from build123d import *

# Parameters (mm, degrees)
SKETCH_1_R      = 1.75
EXTRUDE_1_DEPTH = 1.6
SKETCH_2_W      = 61.5
SKETCH_2_H      = 44.5
EXTRUDE_2_DEPTH = 5.2


with BuildPart() as part:
    # 草图1 → 凸台-拉伸1 (new body)
    with BuildSketch(Plane(origin=(0, 0, 0), x_dir=(1, 0, 0), z_dir=(0, 1, 0))):
        with BuildLine():
            Line((1.5, 0), (73, 0))
            ThreePointArc((73, 0), (74.060660172, 0.439339828), (74.5, 1.5))
            Line((74.5, 1.5), (74.5, 41.5))
            ThreePointArc((74.5, 41.5), (74.060660172, 42.560660172), (73, 43))
            Line((73, 43), (1.5, 43))
            ThreePointArc((1.5, 43), (0.439339828, 42.560660172), (0, 41.5))
            Line((0, 41.5), (0, 1.5))
            ThreePointArc((0, 1.5), (0.439339828, 0.439339828), (1.5, 0))
        make_face()
        with Locations(Location((3.05, 39.85, 0), (0, 0, 270))):
            Circle(SKETCH_1_R, mode=Mode.SUBTRACT)
        with Locations(Location((3.05, 3.15, 0), (0, 0, 270))):
            Circle(SKETCH_1_R, mode=Mode.SUBTRACT)
        with Locations(Location((71.45, 39.85, 0), (0, 0, 270))):
            Circle(SKETCH_1_R, mode=Mode.SUBTRACT)
        with Locations(Location((71.45, 3.15, 0), (0, 0, 270))):
            Circle(SKETCH_1_R, mode=Mode.SUBTRACT)
    extrude(amount=EXTRUDE_1_DEPTH)

    # 草图2 → 凸台-拉伸2 (add)
    with BuildSketch(Plane(origin=(0, 1.6, 0), x_dir=(1, 0, 0), z_dir=(0, 1, 0))):
        with Locations((37.25, 21.5)):
            Rectangle(SKETCH_2_W, SKETCH_2_H)
    extrude(amount=EXTRUDE_2_DEPTH)


solid = part.part
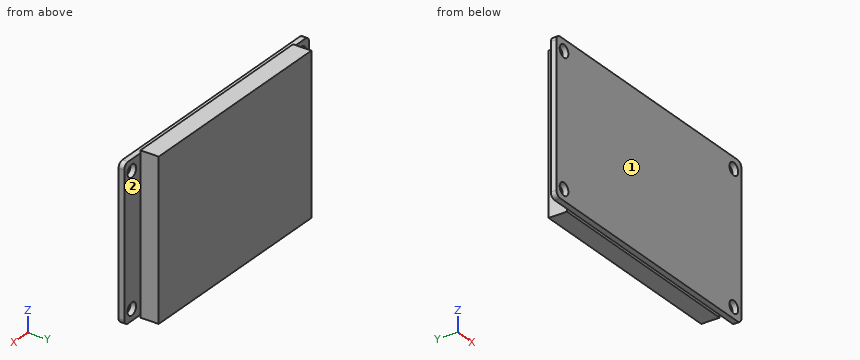
The listing builds one solid part. Answer for the finished solid, in the listing's coordinates (mm). Face numbers are marked on the shaded views. A direction names the side the tool comes from. Give positions to 0.01 mm unless a question says otherwise; leave off trailing zeros. Loops run counter-clockwise (first coordinate to the right, second up) from the corner with the lowest first, then second, coordinate; pieces in that order, holes last. Notation, with made-up numbers: M -9,-18 L 7,-18 A23 ccw 7,21 Z; hole C -23,31.5 d11. An arc over 180 degrees is marked long. Answer as CSV lines item,"result".
Item 1: The part is cut by section D-D (y = 3.5). Give the vertices of the cut face in (x, z).
Values follow:
outline,"M 6.5,-43.75 L 68,-43.75 L 68,0.75 L 6.5,0.75 Z"
Item 2: The part is cut by section C-C (z = -10.5). Give the vertices of the cut face in (x, y), and give its area (3 significant figures).
Values follow:
outline,"M 0,0 L 74.5,0 L 74.5,1.6 L 68,1.6 L 68,6.8 L 6.5,6.8 L 6.5,1.6 L 0,1.6 Z"
area,"439 mm^2"
Item 3: The part is cut by section B-B (x = 71.45). Give the vertices of the cut face in (y, z), and give its area (3 significant figures).
Values follow:
outline,"M 0,-43 L 1.6,-43 L 1.6,-41.6 L 0,-41.6 Z; M 0,-38.1 L 1.6,-38.1 L 1.6,-4.9 L 0,-4.9 Z; M 0,-1.4 L 1.6,-1.4 L 1.6,0 L 0,0 Z"
area,"57.6 mm^2"
Item 4: The part is cut by section A-A (z = -3.15). Give the vertices of the cut face in (x, y).
Values follow:
outline,"M 0,0 L 1.3,0 L 1.3,1.6 L 0,1.6 Z; M 4.8,0 L 69.7,0 L 69.7,1.6 L 68,1.6 L 68,6.8 L 6.5,6.8 L 6.5,1.6 L 4.8,1.6 Z; M 73.2,0 L 74.5,0 L 74.5,1.6 L 73.2,1.6 Z"
Item 5: Given pin 1 Ø4.5 at (x, z) = (71.45, -3.15) entering from +Y; pin 2 Ø0.8 at (x, z) = (48.5, 0.5) entering from -Y; pin 3 Ø3 at (y, z) = (5.5, -33.5) entering from -X; pin 4 Ø3 at (x, z) = (3.05, -3.15) entering from -Y, each flat-ended and moving along its own axis, determine where each tip first touches the part or whether it passes through.
Values follow:
pin 1,"stops at y = 1.6"
pin 2,"stops at y = 1.6"
pin 3,"stops at x = 6.5"
pin 4,"passes through"
Item 6: Which of the six approach directions +Z, -Z, +X, -X, +Y, -Y give full straight-line access (tool end or side, diameter ignored) to the marked faces 1 and 2?
Values follow:
face 1,"+Z, -Z, +X, -X, -Y"
face 2,"+Z, -Z, +X, +Y"
Item 7: Straight lines are drawn through the part: line 1 along X through (y, z) = (0.5, -39.85); line 2 along Z through (x, y) = (71.45, 1.1); line 3 along X through (y, z) = (4.5, -31). For each, find the intervals that lie inside material, in ascending order. Write a range as [from, to].
Values follow:
line 1,"x = [0, 1.3], [4.8, 69.7], [73.2, 74.5]"
line 2,"z = [-43, -41.6], [-38.1, -4.9], [-1.4, 0]"
line 3,"x = [6.5, 68]"
